Verification items for this drawing (mm, ordinates from the low corner). Round coordinates to 2 decimals unless told otherwise and drop trailing zeros. Loops run counter-clockwise (first coordinate to the right, second up) from the corner with the lowest first, then second, coordinate; pieces in that order, holes last. Notation, with made-up numbers: M 25.25,10 L 63.25,10 A22 ccw 63.25,36 Z; hole C 6.25,71.25 d2. An arc over 180 degrees is marked long. Answer in a Markdown table with one row per item. Add a question column.
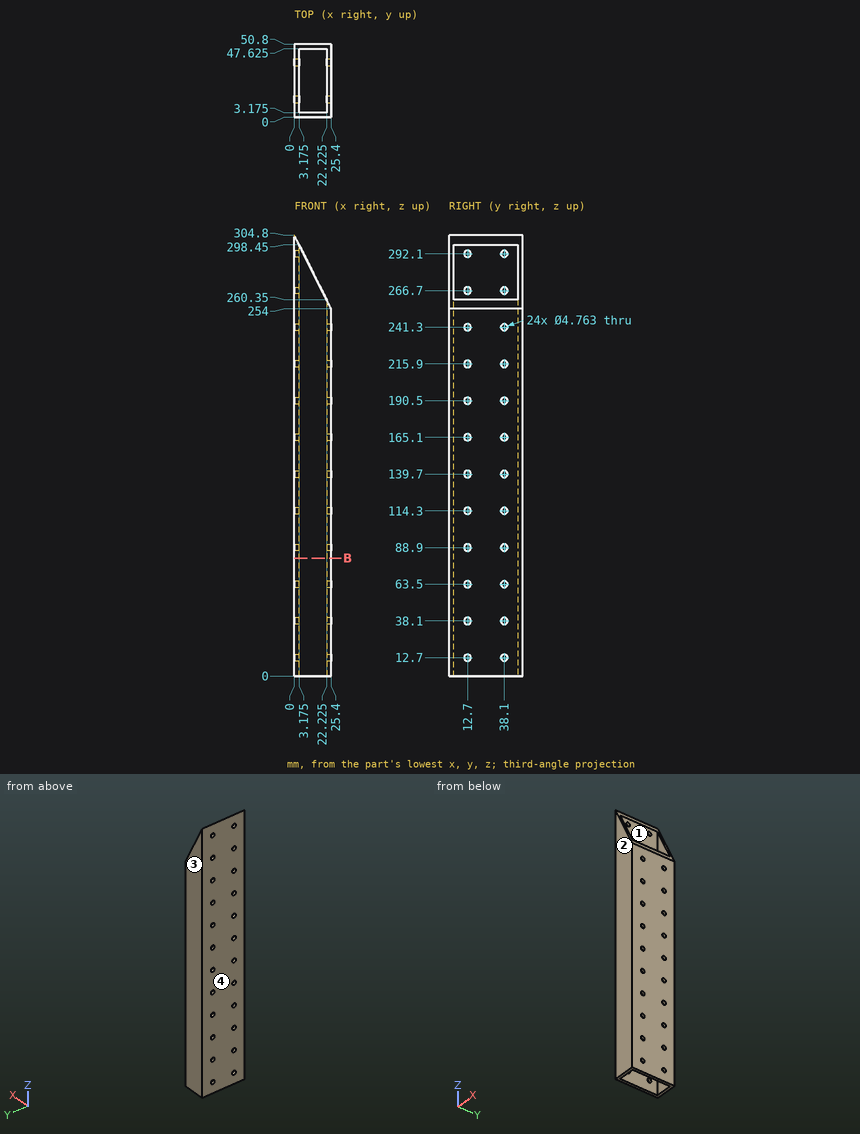
1) Thickness scan on L1, parallel to Y at x = 2.5, z = 190.5; L2, parallel to X at y = 8.5, z = 178.5 (1 decimal); L3, parallel to Y at x = 10.5, z = 149 (1 decimal). Record the ranges inside material, lowest first. Write a range as [from, to].
2) Cross-section at B-B, the plane z = 81.5. Record the boundary of the cut face in (x, y) (1 decimal).
3) Go/stop test with flat-tipped pins: pin 1 (7.5 mm diameter, centred on y = 38.1, z = 241.3, fed in from -X); pin 2 (3 mm diameter, centred on y = 12.7, z = 114.3, fed in from +X). Record where each tip stops, or that it passes through.
4) Draft check along Y on the marked faces 1, 2, 3 and 4. Enter one of: +Y half, -Y half, draft (parallel to the pull), parting line (faces both ways), or undercut.
Worked answers:
| question | item | result |
|---|---|---|
| 1 | L1 | y = [0, 10.32], [15.08, 35.72], [40.48, 50.8] |
| 1 | L2 | x = [0, 3.2], [22.2, 25.4] |
| 1 | L3 | y = [0, 3.2], [47.6, 50.8] |
| 2 | outline | M 0,0 L 25.4,0 L 25.4,50.8 L 0,50.8 Z; hole M 3.2,3.2 L 22.2,3.2 L 22.2,47.6 L 3.2,47.6 Z |
| 3 | pin 1 | stops at x = 0 |
| 3 | pin 2 | passes through |
| 4 | face 1 | undercut |
| 4 | face 2 | -Y half |
| 4 | face 3 | +Y half |
| 4 | face 4 | draft |
